Verification items for the finished model (mm, model axes). Give positions to 0.01 mm unless a question says otherwise; leave off trailing zeros. Write each loop counter-clockwise with the first axis right and the second up, starting at its lowest first coordinate (ties: lowest second). Pieces come first, ordered by that corner, then holes. Notation, with made-up numbers: (9.25, 42.5) -> (17.25, 42.5) arc R20 ccw to (17.25, 57.5) -> close; hole circle Ø6 at (30.25, 64). An arc over 180 degrees is marked (long way). Use one line per item in the form item = value. Start each with the question number.
(1) Section check B-B, the plane x = 9. Record the cut outline in (y, z).
(2) Section check D-D, the plane x = 52. Record the cut outline in (y, z).
(3) Scan lines: L1, parallel to Y at x = 6, z = 0.8; L2, parallel to Y at x = 9.5, z = 2.25; L3, parallel to Y at x = 16, z = 1.4. Record each from-to range of solid material in increasing order.
(4) Section check C-C, the plane y = 16. Record the cut outline in (x, z) (1 decimal), plus the area to 3 significant figures.
from build123d import *

# Parameters (mm, degrees)
F1_DEPTH = 2.38125
F2_R     = 2.38125
F3_DEPTH = 2.38225
F5_DEPTH = 25.4


with BuildPart() as f1:
    # F0 (on Top) → F1 (new body)
    with BuildSketch(Plane.XY):
        with BuildLine():
            Line((60.325, 19.05), (7.9375, 19.05))
            ThreePointArc((7.9375, 19.05), (2.32484, 16.72516), (0, 11.1125))
            Line((0, 11.1125), (0, 0))
            Line((0, 0), (9.525, 0))
            Line((9.525, 0), (12.117365, 7.627166))
            ThreePointArc((12.117365, 7.627166), (13.478615, 9.513592), (15.663196, 10.313094))
            Line((15.663196, 10.313094), (60.325, 12.7))
            Line((60.325, 12.7), (60.325, 19.05))
        make_face()
    extrude(amount=F1_DEPTH)

    # F2 (on face) → F3 (cut, through all)
    with BuildSketch(Plane.XY.offset(2.38125)):
        with Locations((7.9375, 11.1125)):
            Circle(F2_R)
    extrude(amount=-F3_DEPTH, mode=Mode.SUBTRACT)

    # F4 (on face) → F5 (cut)
    with BuildSketch(Plane(origin=(0, 19.05, 0), x_dir=(-1, 0, 0), z_dir=(0, 1, 0))):
        Polygon((-45.61263, 0), (-60.325, 0.79375), (-60.325, 0), align=None)
        Polygon((-45.61263, 2.38125), (-60.325, 2.38125), (-60.325, 1.5875), align=None)
    extrude(amount=-F5_DEPTH, mode=Mode.SUBTRACT)


solid = f1.part
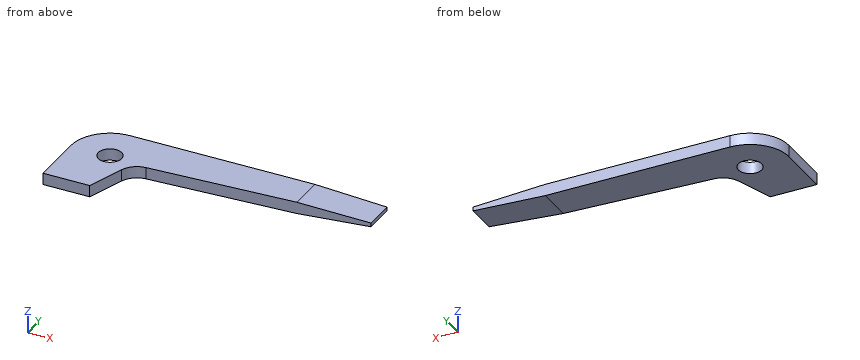
Completed:
q1.outline = (0, 0) -> (8.98, 0) -> (8.98, 2.38) -> (0, 2.38) -> close; (13.24, 0) -> (19.05, 0) -> (19.05, 2.38) -> (13.24, 2.38) -> close
q2.outline = (12.26, 0.34) -> (19.05, 0.34) -> (19.05, 2.04) -> (12.26, 2.04) -> close
q3.L1 = 0 to 9.73, 12.5 to 18.81
q3.L2 = 0 to 9.32, 12.91 to 19.05
q3.L3 = 10.33 to 19.05
q4.outline = (1.7, 0) -> (45.6, 0) -> (60.3, 0.8) -> (60.3, 1.6) -> (45.6, 2.4) -> (1.7, 2.4) -> close
q4.area = 128 mm²
